CAD build for the part. Positions are in the model's coordinates, mm. Face numbers are marked on the shaded views. A direction names the side the tool comes from. Give positions to 0.01 mm unless a question says otherwise; leave off trailing zeros. Loops run counter-clockwise (first coordinate to the right, second up) from the corner with the lowest first, then second, coordinate; pieces in that order, holes last. Notation, with made-up numbers: M -36,48.5 L 14,48.5 A32 ccw 14,74.5 Z; hole C 20.25,53 d2. An arc over 180 degrees is marked long. One line per question, with ' | ' between items.
```python
from build123d import *

# Parameters (mm, degrees)
BOSS_EXTRUDE1_DEPTH   = 1
SKETCH3_R             = 2.6162
BOSS_EXTRUDE1_2_DEPTH = 1
SKETCH4_R             = 2.6162
BOSS_EXTRUDE2_DEPTH   = 1.5
BOSS_EXTRUDE3_DEPTH   = 3
SKETCH6_W             = 15.9258
SKETCH6_H             = 11.25
BOSS_EXTRUDE4_DEPTH   = 5
SKETCH7_W             = 13.5128
SKETCH7_H             = 10
CUT_EXTRUDE1_DEPTH    = 5
CUT_EXTRUDE2_DEPTH    = 5
FILLET1_R             = 2.54
FILLET2_R             = 2.54
FILLET3_R             = 7.62
FILLET4_R             = 1.905


with BuildPart() as part:
    # Sketch3 → Boss-Extrude1 (new body)
    with BuildSketch(Plane(origin=(0, 0, 0), x_dir=(1, 0, 0), z_dir=(0, 1, 0))):
        Polygon((6.7564, 24.25), (6.7564, 20.22), (7.9629, 20.22), (7.9629, 25.5), (-7.9629, 25.5), (-7.9629, 20.22), (-6.7564, 20.22), (-6.7564, 24.25), align=None)
    extrude(amount=BOSS_EXTRUDE1_DEPTH)



with BuildPart() as body_2:
    # Sketch3 → Boss-Extrude1 2 (new body)
    with BuildSketch(Plane(origin=(0, 0, 0), x_dir=(1, 0, 0), z_dir=(0, 1, 0))):
        with BuildLine():
            Line((6.7564, 12.6), (6.7564, 4.876812672))
            ThreePointArc((6.7564, 4.876812672), (6.776225919, 4.847421317), (6.796505263, 4.818340964))
            ThreePointArc((6.796505263, 4.818340964), (0, -8.3312), (-6.796505263, 4.818340964))
            ThreePointArc((-6.796505263, 4.818340964), (-6.776225919, 4.847421317), (-6.7564, 4.876812672))
            Line((-6.7564, 4.876812672), (-6.7564, 12.6))
            Line((-6.7564, 12.6), (-7.9629, 12.6))
            Line((-7.9629, 12.6), (-7.9629, 10.019330915))
            ThreePointArc((-7.9629, 10.019330915), (-8.553832276, 8.174549356), (-10.10666, 7.016470768))
            Line((-10.10666, 7.016470768), (-17.42186, 4.50429022))
            ThreePointArc((-17.42186, 4.50429022), (-20.6375, 0), (-17.42186, -4.50429022))
            Line((-17.42186, -4.50429022), (-3.22159376, -9.380935099))
            ThreePointArc((-3.22159376, -9.380935099), (0, -9.9187), (3.22159376, -9.380935099))
            Line((3.22159376, -9.380935099), (17.42186, -4.50429022))
            ThreePointArc((17.42186, -4.50429022), (20.6375, 0), (17.42186, 4.50429022))
            Line((17.42186, 4.50429022), (10.10666, 7.016470768))
            ThreePointArc((10.10666, 7.016470768), (8.553832276, 8.174549356), (7.9629, 10.019330915))
            Line((7.9629, 10.019330915), (7.9629, 12.6))
            Line((7.9629, 12.6), (6.7564, 12.6))
        make_face()
        with Locations(Location((-15.875, 0, 0), (0, 0, 270))):
            Circle(SKETCH3_R, mode=Mode.SUBTRACT)
        with Locations(Location((15.875, 0, 0), (0, 0, 270))):
            Circle(SKETCH3_R, mode=Mode.SUBTRACT)
    extrude(amount=BOSS_EXTRUDE1_2_DEPTH)


with BuildPart() as part_1:
    add(part.part)

    add(body_2.part)  # Boss-Extrude2 merges body 2
    # Sketch4 → Boss-Extrude2 (add)
    with BuildSketch(Plane(origin=(0, 1, 0), x_dir=(1, 0, 0), z_dir=(0, 1, 0))):
        with BuildLine():
            Line((7.9629, 20.22), (7.9629, 25.5))
            Line((7.9629, 25.5), (-7.9629, 25.5))
            Line((-7.9629, 25.5), (-7.9629, 20.22))
            Line((-7.9629, 20.22), (-7.9629, 12.6))
            Line((-7.9629, 12.6), (-7.9629, 10.019330915))
            ThreePointArc((-7.9629, 10.019330915), (-8.553832276, 8.174549356), (-10.10666, 7.016470768))
            Line((-10.10666, 7.016470768), (-17.42186, 4.50429022))
            ThreePointArc((-17.42186, 4.50429022), (-20.6375, 0), (-17.42186, -4.50429022))
            Line((-17.42186, -4.50429022), (-3.22159376, -9.380935099))
            ThreePointArc((-3.22159376, -9.380935099), (0, -9.9187), (3.22159376, -9.380935099))
            Line((3.22159376, -9.380935099), (17.42186, -4.50429022))
            ThreePointArc((17.42186, -4.50429022), (20.6375, 0), (17.42186, 4.50429022))
            Line((17.42186, 4.50429022), (10.10666, 7.016470768))
            ThreePointArc((10.10666, 7.016470768), (8.553832276, 8.174549356), (7.9629, 10.019330915))
            Line((7.9629, 10.019330915), (7.9629, 12.6))
            Line((7.9629, 12.6), (7.9629, 20.22))
        make_face()
        with Locations(Location((15.875, 0, 0), (0, 0, 270))):
            Circle(SKETCH4_R, mode=Mode.SUBTRACT)
        with Locations(Location((-15.875, 0, 0), (0, 0, 270))):
            Circle(SKETCH4_R, mode=Mode.SUBTRACT)
        with BuildLine():
            Line((-6.7564, 24.25), (6.7564, 24.25))
            Line((6.7564, 24.25), (6.7564, 20.22))
            Line((6.7564, 20.22), (6.7564, 12.6))
            Line((6.7564, 12.6), (6.7564, 4.876812672))
            ThreePointArc((6.7564, 4.876812672), (6.776225919, 4.847421317), (6.796505263, 4.818340964))
            ThreePointArc((6.796505263, 4.818340964), (0, -8.3312), (-6.796505263, 4.818340964))
            ThreePointArc((-6.796505263, 4.818340964), (-6.776225919, 4.847421317), (-6.7564, 4.876812672))
            Line((-6.7564, 4.876812672), (-6.7564, 12.6))
            Line((-6.7564, 12.6), (-6.7564, 20.22))
            Line((-6.7564, 20.22), (-6.7564, 24.25))
        make_face(mode=Mode.SUBTRACT)
    extrude(amount=BOSS_EXTRUDE2_DEPTH)

    # Sketch5 → Boss-Extrude3 (add)
    # profile 1 of 2: a face of its own
    with BuildSketch(Plane(origin=(0, 2.5, 0), x_dir=(1, 0, 0), z_dir=(0, 1, 0))):
        with BuildLine():
            Line((-10.10666, 7.016470768), (-9.91527155, -0.260767662))
            ThreePointArc((-9.91527155, -0.260767662), (-7.996166023, -5.868725468), (-3.22159376, -9.380935099))
            ThreePointArc((-3.22159376, -9.380935099), (0, -9.9187), (3.22159376, -9.380935099))
            ThreePointArc((3.22159376, -9.380935099), (7.996166023, -5.868725468), (9.91527155, -0.260767662))
            Line((9.91527155, -0.260767662), (10.10666, 7.016470768))
            ThreePointArc((10.10666, 7.016470768), (8.553832276, 8.174549356), (7.9629, 10.019330915))
            Line((7.9629, 10.019330915), (7.9629, 25.5))
            Line((7.9629, 25.5), (-7.9629, 25.5))
            Line((-7.9629, 25.5), (-7.9629, 10.019330915))
            ThreePointArc((-7.9629, 10.019330915), (-8.553832276, 8.174549356), (-10.10666, 7.016470768))
        make_face()
        with BuildLine():
            Line((-6.7564, 4.876812672), (-6.7564, 24.25))
            Line((-6.7564, 24.25), (6.7564, 24.25))
            Line((6.7564, 24.25), (6.7564, 4.876812672))
            ThreePointArc((6.7564, 4.876812672), (6.776225919, 4.847421317), (6.796505263, 4.818340964))
            ThreePointArc((6.796505263, 4.818340964), (0, -8.3312), (-6.796505263, 4.818340964))
            ThreePointArc((-6.796505263, 4.818340964), (-6.776225919, 4.847421317), (-6.7564, 4.876812672))
        make_face(mode=Mode.SUBTRACT)
    # profile 2 of 2: a face of its own
    with BuildSketch(Plane(origin=(0, 2.5, 0), x_dir=(1, 0, 0), z_dir=(0, 1, 0))):
        with BuildLine():
            ThreePointArc((-6.796505263, 4.818340964), (-6.776225919, 4.847421317), (-6.7564, 4.876812672))
            Line((-6.7564, 4.876812672), (-6.7564, 24.25))
            Line((-6.7564, 24.25), (6.7564, 24.25))
            Line((6.7564, 24.25), (6.7564, 4.876812672))
            ThreePointArc((6.7564, 4.876812672), (6.776225919, 4.847421317), (6.796505263, 4.818340964))
            ThreePointArc((6.796505263, 4.818340964), (0, -8.3312), (-6.796505263, 4.818340964))
        make_face()
    extrude(amount=BOSS_EXTRUDE3_DEPTH)

    # Sketch6 → Boss-Extrude4 (add)
    with BuildSketch(Plane(origin=(0, 5.5, 0), x_dir=(1, 0, 0), z_dir=(0, 1, 0))):
        with Locations((0, 19.875)):
            Rectangle(SKETCH6_W, SKETCH6_H)
    extrude(amount=BOSS_EXTRUDE4_DEPTH)

    # Sketch7 → Cut-Extrude1 (cut)
    with BuildSketch(Plane.XZ.offset(-2.5)):
        with Locations((0, -19.25)):
            Rectangle(SKETCH7_W, SKETCH7_H)
    extrude(amount=-CUT_EXTRUDE1_DEPTH, mode=Mode.SUBTRACT)

    # Sketch8 → Cut-Extrude2 (cut)
    with BuildSketch(Plane.ZY.offset(7.9629)):
        Polygon((-16.25, 7.5), (-16.25, 1), (-14.25, 1), (-14.25, 5.5), (-14.25, 7.5), align=None)
    extrude(amount=-CUT_EXTRUDE2_DEPTH, mode=Mode.SUBTRACT)

    # Fillet1
    fillet1_edges = [part_1.edges().sort_by_distance(p)[0] for p in [
        (-6.7564, 1.25, -4.876812672),
    ]]
    fillet(fillet1_edges, radius=FILLET1_R)

    # Fillet2
    fillet2_edges = [part_1.edges().sort_by_distance(p)[0] for p in [
        (6.7564, 1.25, -4.876812672),
    ]]
    fillet(fillet2_edges, radius=FILLET2_R)

    # Fillet3
    fillet3_edges = [part_1.edges().sort_by_distance(p)[0] for p in [
        (10.10666, 4, -7.016470768),
        (-10.10666, 4, -7.016470768),
    ]]
    fillet(fillet3_edges, radius=FILLET3_R)

    # Fillet4
    fillet4_edges = [part_1.edges().sort_by_distance(p)[0] for p in [
        (-7.9629, 5.25, -25.5),
        (7.9629, 5.25, -25.5),
    ]]
    fillet(fillet4_edges, radius=FILLET4_R)


solid = part_1.part
```
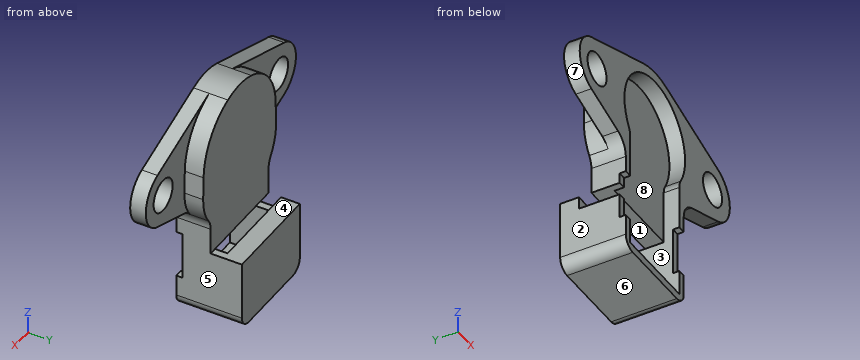
Item 1: 3-axis set-ups, long thin cutter, end or side, ignore diameter. For the marked faces 1, 2, 3, 4 and 5: which of +Z, -Z, +X, -X, +Y, -Y reach the whole face in a straight line?
Conclusion:
face 1: -X, -Y | face 2: -Z, -X, +Y, -Y | face 3: -Y | face 4: +Z, +X, -X, +Y | face 5: -Z, +X, +Y, -Y
Item 2: Saw through at D-D on z = -21.5. Give the cut face in (x, y), and give its area (3 significant figures).
Conclusion:
outline: M -7.96,0 L -6.76,0 L -6.76,7.5 L 6.76,7.5 L 6.76,0 L 7.96,0 L 7.96,10.5 L -7.96,10.5 Z | area: 65.9 mm²
Item 3: Mould opens along X. For the marked faces 6, 7 and 8 say: pulls with the +X half, pulls with the -X half, needs draft (parallel to the pull), parting line crosses it, or undercut.
Conclusion:
face 6: needs draft | face 7: pulls with the -X half | face 8: undercut
Item 4: Saw through at A-A on x = 0. Give the cut face in (y, z).
Conclusion:
outline: M 0,-25.5 L 10.5,-25.5 L 10.5,-14.25 L 7.5,-14.25 L 7.5,-24.25 L 0,-24.25 Z; M 0,8.33 L 2.5,8.33 L 2.5,-14.25 L 5.5,-14.25 L 5.5,9.92 L 0,9.92 Z
Item 5: Saw through at B-B on y = 3. Give the cut face in (x, z) (3 decimals).
Conclusion:
outline: M -10.014,-3.485 A7.62 ccw -8.567,-8.156 A3.175 cw -7.963,-10.019 L -7.963,-14.25 L 6.756,-14.25 L 6.756,-24.25 L -6.756,-24.25 L -6.756,-16.25 L -7.963,-16.25 L -7.963,-23.595 A1.905 ccw -6.058,-25.5 L 6.058,-25.5 A1.905 ccw 7.963,-23.595 L 7.963,-10.019 A3.175 cw 8.567,-8.156 A7.62 ccw 10.014,-3.485 L 9.915,0.261 A9.919 ccw -9.915,0.261 Z
Item 6: Drop flat-ended pins along their axis: P1, Ø1, axis at x = -7.5, z = -19, coming from the -Y side; P2, Ø2, axis at y = 3.5, z = -12, coming from the -X side; P3, Ø19, axis at x = -9.5, z = 1, coming from the +Y side; P4, Ø8, axis at x = -12, z = -4, coming from the -Y side. Give the stop position or say it passes through.
Conclusion:
P1: y = 1 | P2: x = -7.96 | P3: y = 5.5 | P4: y = 0
Item 7: Drill centre lines: line 1 along X through (y, z) = (0.75, 0); line 2 along Z through (x, y) = (0, 1.4); line 3 along X through (y, z) = (5.5, -20.5). Where is each one in solid material? Low to high. Write a range as [from, to].
Conclusion:
line 1: [-20.64, -18.49], [-13.26, -8.33], [8.33, 13.26], [18.49, 20.64] | line 2: [-25.5, -24.25], [8.33, 9.92] | line 3: [-7.96, -6.76], [6.76, 7.96]
Item 8: Saw through at C-C on z = -0.5. Give the cut face in (x, y).
Conclusion:
outline: M -20.61,0 L -18.44,0 L -18.44,2.5 L -20.61,2.5 Z; M -13.31,0 L -8.32,0 L -8.32,2.5 L 8.32,2.5 L 8.32,0 L 13.31,0 L 13.31,2.5 L 9.94,2.5 L 9.94,5.5 L -9.94,5.5 L -9.94,2.5 L -13.31,2.5 Z; M 18.44,0 L 20.61,0 L 20.61,2.5 L 18.44,2.5 Z
